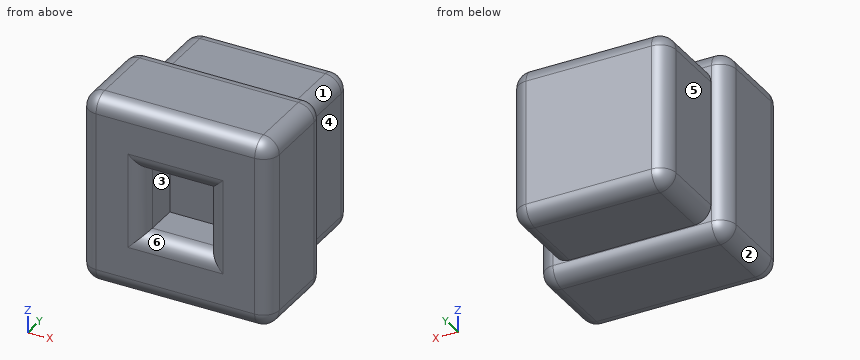
```python
from build123d import *

# Parameters (mm, degrees)
SKETCH1_W           = 9.9
SKETCH1_H           = 9.9
BOSS_EXTRUDE1_DEPTH = 5
SKETCH2_W           = 12
SKETCH2_H           = 12
BOSS_EXTRUDE2_DEPTH = 6
SKETCH3_W           = 4
SKETCH3_H           = 4
CUT_EXTRUDE1_DEPTH  = 3
FILLET1_R           = 1


with BuildPart() as part:
    # Sketch1 → Boss-Extrude1 (new body)
    with BuildSketch(Plane(origin=(0, 0, 0), x_dir=(1, 0, 0), z_dir=(0, 1, 0))):
        Rectangle(SKETCH1_W, SKETCH1_H)
    extrude(amount=BOSS_EXTRUDE1_DEPTH)

    # Sketch2 → Boss-Extrude2 (add)
    with BuildSketch(Plane.XZ):
        Rectangle(SKETCH2_W, SKETCH2_H)
    extrude(amount=BOSS_EXTRUDE2_DEPTH)

    # Sketch3 → Cut-Extrude1 (cut)
    with BuildSketch(Plane.XZ.offset(6)):
        Rectangle(SKETCH3_W, SKETCH3_H)
    extrude(amount=-CUT_EXTRUDE1_DEPTH, mode=Mode.SUBTRACT)

    # Fillet1
    fillet1_edges = [part.edges().sort_by_distance(p)[0] for p in [
        (4.95, 5, 0),
        (6, 0, 0),
        (6, -3, -6),
        (0, 0, 6),
        (6, -3, 6),
        (-6, 0, 0),
        (-6, -3, 6),
        (0, 0, -6),
        (-6, -3, -6),
        (6, -6, 0),
        (0, -6, 6),
        (-6, -6, 0),
        (0, -6, -6),
        (0, 5, -4.95),
        (-2, -6, 0),
        (0, -6, -2),
        (2, -6, 0),
        (0, -6, 2),
        (-4.95, 5, 0),
        (-4.95, 2.5, -4.95),
        (4.95, 2.5, -4.95),
        (4.95, 2.5, 4.95),
        (-4.95, 2.5, 4.95),
        (0, 5, 4.95),
    ]]
    fillet(fillet1_edges, radius=FILLET1_R)


solid = part.part
```
Here's how the part is built. I have some questions about the finished solid (model axes, mm). Face numbers are marked on the shaded views. A direction names the side the tool comes from. Coordinates: 2 decimals unless noted, no trailing zeros. Write each loop counter-clockwise with the first axis right and the second up, starting at its lowest first coordinate (ties: lowest second). Pieces come first, ordered by that corner, then holes. Notation, with made-up numbers: (-27.5, 38) -> (26.5, 38) arc R28 ccw to (26.5, 56) -> close; hole circle Ø10 at (9.5, 55). An arc over 180 degrees is marked (long way). Use a Markdown table: item, result. Add a question column.
(1) If we section it at D-D, the plane z = -0.5: Write out the boundary of the cut face in (x, y).
(2) Please list where these lines run through material, in increasing order: line 1 (X direction, y = -4.75, z = -0.75); line 2 (Z direction, x = 4, y = 4).
(3) We'd pull the mould along Z, two halves only. Please class the marked faces 1, 2 and 3: +Z half, -Z half, draft (parallel to the pull), parting line (faces both ways), or undercut.
(4) If we section it at C-C, the plane y = 1.75: Write out the boundary of the cut face in (x, z).
(5) For the marked faces 4, 5 and 6, which set-ups out of +Z, -Z, +X, -X, +Y, -Y let a thin tool reach every point of the face, with its end or its side?
(6) If we section it at A-A, the plane y = -4.5: Write out the boundary of the cut face in (x, z), and give its area (3 significant figures).
(7) I'm going to push flat-ended pins straight in: P1, Ø3, axis at x = 0, z = -1, coming from the -Y side; P2, Ø3, axis at y = 2.5, z = -1.5, coming from the -X side; P3, Ø3, axis at x = -1, y = 2, coming from the +Z side. Where does each tip first touch, or does it pass through?
(8) If we section it at B-B, the plane x = 1: Write out the boundary of the cut face in (y, z).
Outcome:
| question | item | result |
|---|---|---|
| 1 | outline | (-6, -5) arc R1 ccw to (-5, -6) -> (-3, -6) arc R1 ccw to (-2, -5) -> (-2, -3) -> (2, -3) -> (2, -5) arc R1 ccw to (3, -6) -> (5, -6) arc R1 ccw to (6, -5) -> (6, -1) arc R1 ccw to (5, 0) -> (4.95, 0) -> (4.95, 4) arc R1 ccw to (3.95, 5) -> (-3.95, 5) arc R1 ccw to (-4.95, 4) -> (-4.95, 0) -> (-5, 0) arc R1 ccw to (-6, -1) -> close |
| 2 | line 1 | x = -6 to -2, 2 to 6 |
| 2 | line 2 | z = -4.95 to 4.95 |
| 3 | face 1 | +Z half |
| 3 | face 2 | -Z half |
| 3 | face 3 | undercut |
| 4 | outline | (-4.95, -3.95) arc R1 ccw to (-3.95, -4.95) -> (3.95, -4.95) arc R1 ccw to (4.95, -3.95) -> (4.95, 3.95) arc R1 ccw to (3.95, 4.95) -> (-3.95, 4.95) arc R1 ccw to (-4.95, 3.95) -> close |
| 5 | face 4 | +Z, -Z, +X, +Y |
| 5 | face 5 | +Z, -Z, -X, +Y |
| 5 | face 6 | -Y |
| 6 | outline | (-6, -5) arc R1 ccw to (-5, -6) -> (5, -6) arc R1 ccw to (6, -5) -> (6, 5) arc R1 ccw to (5, 6) -> (-5, 6) arc R1 ccw to (-6, 5) -> close; hole (-2, -2) -> (2, -2) -> (2, 2) -> (-2, 2) -> close |
| 6 | area | 127 mm^2 |
| 7 | P1 | stops at y = -5.87 |
| 7 | P2 | stops at x = -4.95 |
| 7 | P3 | stops at z = 4.95 |
| 8 | outline | (-6, -5) arc R1 ccw to (-5, -6) -> (-1, -6) arc R1 ccw to (0, -5) -> (0, -4.95) -> (4, -4.95) arc R1 ccw to (5, -3.95) -> (5, 3.95) arc R1 ccw to (4, 4.95) -> (0, 4.95) -> (0, 5) arc R1 ccw to (-1, 6) -> (-5, 6) arc R1 ccw to (-6, 5) -> (-6, 3) arc R1 ccw to (-5, 2) -> (-3, 2) -> (-3, -2) -> (-5, -2) arc R1 ccw to (-6, -3) -> close |
